Build history of the part. All positions in model axes, mm. Give positions to 0.01 mm unless a question says otherwise; leave off trailing zeros. Loops run counter-clockwise (first coordinate to the right, second up) from the corner with the lowest first, then second, coordinate; pieces in that order, holes last. Notation, with made-up numbers: M 61.5,89.5 L 110.5,89.5 A29 ccw 110.5,127.5 Z; hole C -27,61 d4. An arc over 180 degrees is marked long. Answer as a JSON object with one key per item and string values. Group by question number.
1. Drill centre lines: line 1 along Y through (x, z) = (12, 1.3); line 2 along X through (y, z) = (-0.25, 1.8); line 3 along X through (y, z) = (-2.5, 0.7). Where is each one in solid material? Low to high. Write a range as [from, to].
2. Slice it at A-A (x = 22.5). List the corners of the cut face in (y, z).
3. Drop flat-ended pins along their axis: pin 1 Ø0.6 at (y, z) = (-0.5, 1) entering from +X; pin 2 Ø0.5 at (x, z) = (0, 1) entering from -Y. Give the stop position or say it passes through.
4. Slice it at B-B (x = 6.5). List the corners of the cut face in (y, z), then the cut area to 3 significant figures.
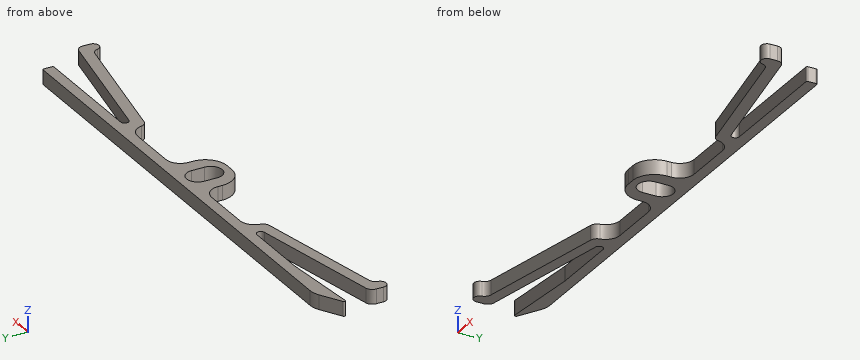
from build123d import *

# Parameters (mm, degrees)
FLAT_DEPTH              = 2
SKETCH3_W               = 7.1
SKETCH3_H               = 7.1
BOSS_EXTRUDE3_DEPTH     = 2
CUT_EXTRUDE1_DEPTH      = 38.889997963
CUT_EXTRUDE1_DEPTH_BACK = 38.889997963
BOSS_EXTRUDE5_DEPTH     = 2
FILLET3_R               = 1
FILLET4_R               = 2
FILLET8_R               = 2
FILLET6_R               = 0.2
FILLET7_R               = 3


with BuildPart() as part:
    # Sketch2 → flat (new body)
    with BuildSketch(Plane.XY):
        Polygon((-32.834936491, 0), (32.834936491, 0), (32.834936491, -1.5), (-25.735011207, -1.5), (-37.165063509, -2.5), align=None)
    extrude(amount=FLAT_DEPTH)

    # Sketch3 → Boss-Extrude3 (add)
    with BuildSketch(Plane(origin=(0, 0, 0), x_dir=(-1, 0, 0), z_dir=(0, 0, -1))):
        with Locations((0, -3.55)):
            Rectangle(SKETCH3_W, SKETCH3_H)
    extrude(amount=-BOSS_EXTRUDE3_DEPTH)

    # Sketch4 → Cut-Extrude1 (cut, two sides: drawn at the far end of the back side and taken through both)
    with BuildSketch(Plane.XY.offset(2).offset(-CUT_EXTRUDE1_DEPTH_BACK)):
        with BuildLine():
            Line((-1.55, -2.75), (-1.55, -4.55))
            ThreePointArc((-1.55, -4.55), (0, -6.1), (1.55, -4.55))
            Line((1.55, -4.55), (1.55, -2.75))
            ThreePointArc((1.55, -2.75), (0, -1.2), (-1.55, -2.75))
        make_face()
    extrude(amount=CUT_EXTRUDE1_DEPTH + CUT_EXTRUDE1_DEPTH_BACK, mode=Mode.SUBTRACT)

    # Sketch6 → Boss-Extrude5 (add)
    with BuildSketch(Plane.XY.offset(2)):
        with BuildLine():
            Line((-16.409257503, -2.585457858), (-35.604897729, -6.278480095))
            Line((-35.604897729, -6.278480095), (-35.604897729, -8.1))
            ThreePointArc((-35.604897729, -8.1), (-34.804897729, -8.9), (-34.004897729, -8.1))
            Line((-34.004897729, -8.1), (-34.004897729, -7.6))
            Line((-34.004897729, -7.6), (-14.365063509, -3.821519905))
            Line((-14.365063509, -3.821519905), (-14.365063509, -1.5))
            Line((-14.365063509, -1.5), (-16.512723649, -1.5))
            ThreePointArc((-16.512723649, -1.5), (-15.96753469, -1.995692576), (-16.409257503, -2.585457858))
        make_face()
    boss_extrude5 = extrude(amount=-BOSS_EXTRUDE5_DEPTH)

    # Mirror4: Boss-Extrude5 across plane
    add(boss_extrude5.mirror(Plane(origin=(0, 0, 0), x_dir=(0, 0, 1), z_dir=(1, 0, 0))))

    # Fillet3
    fillet3_edges = [part.edges().sort_by_distance(p)[0] for p in [
        (-35.604897729, -6.278480095, 1),
        (-34.004897729, -7.6, 1),
        (-14.365063509, -3.821519905, 1),
        (35.604897729, -6.278480095, 1),
        (34.004897729, -7.6, 1),
        (14.365063509, -3.821519905, 1),
    ]]
    fillet(fillet3_edges, radius=FILLET3_R)

    # Fillet4
    fillet4_edges = [part.edges().sort_by_distance(p)[0] for p in [
        (-14.365063509, -1.5, 1),
        (14.365063509, -1.5, 1),
    ]]
    fillet(fillet4_edges, radius=FILLET4_R)

    # Fillet8
    fillet8_edges = [part.edges().sort_by_distance(p)[0] for p in [
        (-3.55, -1.5, 1),
        (3.55, -1.5, 1),
    ]]
    fillet(fillet8_edges, radius=FILLET8_R)

    # Fillet6
    fillet6_edges = [part.edges().sort_by_distance(p)[0] for p in [
        (32.834936491, 0, 1),
        (32.834936491, -1.5, 1),
        (-37.165063509, -2.5, 1),
    ]]
    fillet(fillet6_edges, radius=FILLET6_R)

    # Fillet7
    # the kernel refuses this fillet: 3 mm, written as the material it adds along each edge
    with BuildSketch(Plane(origin=(-25.735011207, -1.5, 0), x_dir=(-0.996194698091746, -0.0871557427476529, 0), z_dir=(0, 0, 1))) as fillet7_piece_1:
        with BuildLine():
            CenterArc((FILLET7_R * 0.0436609429085, FILLET7_R), FILLET7_R, 265, 5)
            Line((-FILLET7_R * 0.0434947998391, FILLET7_R * 0.00380530190825), (0, 0))
            Line((0, 0), (FILLET7_R * 0.0436609429085, 0))
        make_face()
    extrude(amount=2)
    # the kernel refuses this fillet: 3 mm, written as the material it takes off along each edge
    with BuildSketch(Plane(origin=(3.55, -7.1, -7.5), x_dir=(0, 1, 0), z_dir=(0, 0, 1)), Plane(origin=(-3.55, -7.1, -7.5), x_dir=(1, 0, 0), z_dir=(0, 0, 1))) as fillet7_2_piece_1:
        with BuildLine():
            CenterArc((FILLET7_R, FILLET7_R), FILLET7_R, 180, 90)
            Line((0, FILLET7_R), (0, 0))
            Line((0, 0), (FILLET7_R, 0))
        make_face()
    extrude(amount=17, mode=Mode.SUBTRACT)
    with BuildSketch(Plane(origin=(-32.834936491, 0, -2.009618943), x_dir=(1, 0, 0), z_dir=(0, 0, 1))) as fillet7_2_piece_2:
        with BuildLine():
            CenterArc((FILLET7_R * 0.267949192431, -FILLET7_R), FILLET7_R, 90, 30)
            Line((-FILLET7_R * 0.232050807569, -FILLET7_R * 0.133974596216), (0, 0))
            Line((0, 0), (FILLET7_R * 0.267949192431, 0))
        make_face()
    extrude(amount=6.019237886, mode=Mode.SUBTRACT)


solid = part.part
Established:
{
 "1": {"line 1": "y = [-1.5, 0]", "line 2": "x = [-33.23, 32.83]", "line 3": "x = [-16.2, -14.14], [-3.82, -1.53], [1.53, 3.82], [14.14, 16.2]"},
 "2": {"outline": "M -5.39,0 L -3.76,0 L -3.76,2 L -5.39,2 Z; M -1.5,0 L 0,0 L 0,2 L -1.5,2 Z"},
 "3": {"pin 1": "stops at x = 32.83", "pin 2": "stops at y = -7.1"},
 "4": {"outline": "M -1.5,0 L 0,0 L 0,2 L -1.5,2 Z", "area": "3.00 mm^2"}
}
